For this review, take the finished solid that the model builds, in its own axes (mm). A direction names the side the tool comes from. Round coordinates to 2 decimals unless told otherwise and drop trailing zeros. Order: outer loops, then holes, each group sorted by start corner. A loop starts at its lowest first (then second) coordinate and runs counter-clockwise, first axis right, second up. Notation, with made-up numbers: (8.25, 58.25) - (50.25, 58.25) arc R11 cw to (50.25, 70.25) - close; hole circle Ø10 at (-18, 47). An arc over 180 degrees is marked (long way). One line per item, written item: value.
```python
from build123d import *

# Parameters (mm, degrees)
F1_DEPTH = 25
F2_R     = 4.75
F3_DEPTH = 51.2
F5_DEPTH = 20.8
F6_R     = 2.931006
F7_DEPTH = 45.7


with BuildPart() as f1:
    # F0 (on Front) → F1 (new body)
    with BuildSketch(Plane.XZ):
        with BuildLine():
            Line((-46.805558, 22.916667), (-46.805558, 12.916667))
            Line((-46.805558, 12.916667), (-43.568752, 12.916667))
            ThreePointArc((-43.568752, 12.916667), (-38.568828, 17.889121), (-33.568904, 12.916667))
            Line((-33.568904, 12.916667), (-29.305557, 12.916667))
            Line((-29.305557, 12.916667), (0, 12.916667))
            ThreePointArc((0, 12.916667), (5, 17.916667), (10, 12.916667))
            Line((10, 12.916667), (16.527779, 12.916667))
            Line((16.527779, 12.916667), (16.527779, 22.916667))
            Line((16.527779, 22.916667), (8.472223, 22.916667))
            Line((8.472223, 22.916667), (-0.13889, 29.02778))
            Line((-0.13889, 29.02778), (-29.305557, 29.02778))
            Line((-29.305557, 29.02778), (-35.694448, 22.916667))
            Line((-35.694448, 22.916667), (-46.805558, 22.916667))
        make_face()
        with BuildLine():
            ThreePointArc((-33.568904, 12.916667), (-38.568828, 17.889121), (-43.568752, 12.916667))
            ThreePointArc((-43.568752, 12.916667), (-38.582602, 7.88914), (-33.568828, 12.889121))
            ThreePointArc((-33.568828, 12.889121), (-33.568847, 12.902894), (-33.568904, 12.916667))
        make_face()
        with BuildLine():
            ThreePointArc((10, 12.916667), (5, 17.916667), (0, 12.916667))
            ThreePointArc((0, 12.916667), (5, 7.916667), (10, 12.916667))
        make_face()
    extrude(amount=F1_DEPTH)

    # F2 (on Right) → F3 (cut, symmetric)
    with BuildSketch(Plane.YZ):
        with Locations((-13.057046, 18.02115)):
            Circle(F2_R)
    extrude(amount=F3_DEPTH, both=True, mode=Mode.SUBTRACT)

    # F4 (on Right) → F5 (join)
    with BuildSketch(Plane.YZ):
        Polygon((0, 23.411883), (-24.079781, 23.172596), (-24.079781, 13.592975), (-21.914035, 13.598205), (0, 13.65112), align=None)
    extrude(amount=F5_DEPTH)

    # F6 (on Right) → F7 (cut)
    with BuildSketch(Plane.YZ):
        with Locations((-11.352646, 18.537864)):
            Circle(F6_R)
    extrude(amount=F7_DEPTH, mode=Mode.SUBTRACT)


solid = f1.part
```
Item 1: For P1, Ø2, axis at x = 12.5, y = -11.5, coming from the -Z side; P2, Ø2, axis at y = -11.5, z = 10.5, coming from the +X side; P3, Ø0.5, axis at x = 14, y = -24.5, coming from the +Z side; P4, Ø3, axis at y = -12, z = 19.5, coming from the +X side, all flat-tipped, find the tip position at first contact; note any pin that passes through.
Returned:
P1: z = 12.92
P2: x = 9.8
P3: z = 22.92
P4: through
Item 2: Machinability: for faces 1 (the flat face through (-32.455, -12.325, 26.015)), 2 (the flat face through (13, -12, 12.917)), 3 (the flat face through (0, -14.2, 17.2)), 4 (the flat face through (-17, -12, 12.917)), 5 (the flat face through (-45, -12, 12.917)), which of the approach directions +Z, -Z, +X, -X, +Y, -Y give a long, thin tool a straight path to every point of the face, cutting with its end or side? Answer none if there is none.
Returned:
face 1: +Z, -X, +Y, -Y
face 2: -Z, +X, +Y, -Y
face 3: -X
face 4: -Z, +Y, -Y
face 5: -Z, -X, +Y, -Y
Item 3: Take a section at A-A (z = 11.5). Write out the cut boundary in (x, y).
Returned:
outline: (-43.37, -25) - (-33.77, -25) - (-33.77, 0) - (-43.37, 0) - close; (0.2, -25) - (9.8, -25) - (9.8, 0) - (0.2, 0) - close
Item 4: The part is to be moulded in two halves that separate along Z. For faces 6 (the flat face through (-16, -25, 19)), 7 (the flat face through (-41, -12, 22.917)), 8 (the cylindrical face through (10.254, -11.988, 15.677)), 9 (the cylindrical face through (-21.733, -14.087, 13.384)), say which applies: +Z half, -Z half, draft (parallel to the pull), parting line (faces both ways), or undercut.
Returned:
face 6: draft
face 7: +Z half
face 8: undercut
face 9: undercut
Item 5: Take a section at D-D (x = -27). Write out the cut boundary in (y, z).
Returned:
outline: (-25, 12.92) - (0, 12.92) - (0, 29.03) - (-25, 29.03) - close; hole circle Ø9.5 at (-13.06, 18.02)
Item 6: Wall thickness on line 1 (Z direction, x = -8.5, y = -8); line 2 (Z direction, x = -14, y = -13.25); line 3 (X direction, y = -2.5, z = 9.25): over which ranges is each line inside the solid? List them lowest first.
Returned:
line 1: 12.92 to 29.03
line 2: 12.92 to 13.28, 22.77 to 29.03
line 3: -42 to -35.14, 1.6 to 8.4
Item 7: Take a section at B-B (x = 5). Write out the cut boundary in (y, z), plus the area to 3 significant figures.
Returned:
outline: (-25, 7.92) - (0, 7.92) - (0, 25.38) - (-25, 25.38) - close; hole (-14.83, 13.62) arc R4.75 ccw to (-11.26, 13.62) - close; hole circle Ø5.86 at (-11.35, 18.54)
area: 409 mm^2
